Geometry check sheet. Reference: the model listing, model coordinates, mm. Face numbers are marked on the shaded views. A direction names the side the tool comes from. Coordinates: 2 decimals unless noted, no trailing zeros. Loops run counter-clockwise (first coordinate to the right, second up) from the corner with the lowest first, then second, coordinate; pieces in that order, holes last.
Solid Edge part; units mm, degrees
sketch "Sketch1" plane through (0, 0, 0) normal (0, -1, 0) x (1, 0, 0)
  line L0 (0, 25) -> (-95, 25)
  line L1 (-95, 25) -> (-95, 10)
  line L2 (-95, 10) -> (-45, 10)
  line L3 (-45, 10) -> (-45, -10)
  line L4 (-45, -10) -> (-95, -10)
  line L5 (-95, -10) -> (-95, -25)
  line L6 (-95, -25) -> (0, -25)
  arc A0 (0, 25) -> (0, -25) centre (0, 0) cw
  circle A1 centre (0, 0) radius 12.5
extrude "Protrusion1" add sketch "Sketch1" against normal blind 50
sketch "Sketch2" plane through (-47.5, 25, 25) normal (0, 0, 1) x (1, 0, 0)
  line L0 (-22.5, 25) -> (72.5, 25)
  line L1 (72.5, 25) -> (72.5, 10)
  line L2 (72.5, 10) -> (22.5, 10)
  line L3 (22.5, 10) -> (22.5, -10)
  line L4 (22.5, -10) -> (72.5, -10)
  line L5 (72.5, -10) -> (72.5, -25)
  line L6 (72.5, -25) -> (-22.5, -25)
  arc A0 (-22.5, -25) -> (-22.5, 25) centre (-22.5, 0) cw
  circle A1 centre (-22.5, 0) radius 12.5
extrude "ExtrudedProtrusion_2" add sketch "Sketch2" against normal blind 50
fillet "Round_2" radius 25 8 edges at (25, 42.5, 25) (25, 7.5, 25) (25, 42.5, -25) (25, 7.5, -25) (-95, 50, 17.5) (-95, 50, -17.5) (-95, 0, 17.5) (-95, 0, -17.5)
sketch "Sketch3" plane through (-22.5, 0, 0) normal (0, -1, 0) x (-1, 0, 0)
  circle A0 centre (-22.578, 0) radius 12.5
extrude "ExtrudedCutout_1" cut sketch "Sketch3" against normal blind 50
sketch "Sketch4" plane through (-47.5, 25, 25) normal (0, 0, 1) x (-1, 0, 0)
  circle A0 centre (22.5, 0) radius 12.5
extrude "ExtrudedCutout_2" cut sketch "Sketch4" against normal blind 50
sketch "Sketch5" plane through (-47.5, 25, 25) normal (0, 0, 1) x (-1, 0, 0)
  line L0 (-22.5, 10) -> (-72.5, 10)
  line L1 (-72.5, 10) -> (-72.5, -10)
  line L2 (-72.5, -10) -> (-22.5, -10)
  line L3 (-22.5, -10) -> (-22.5, 10)
extrude "ExtrudedCutout_3" cut sketch "Sketch5" against normal blind 50
sketch "Sketch6" plane through (-22.5, 0, 0) normal (0, -1, 0) x (0, 0, -1)
  line L0 (-10, -72.5) -> (10, -72.5)
  line L1 (10, -72.5) -> (10, -22.5)
  line L2 (10, -22.5) -> (-10, -22.5)
  line L3 (-10, -22.5) -> (-10, -72.5)
extrude "ExtrudedCutout_4" cut sketch "Sketch6" against normal blind 50
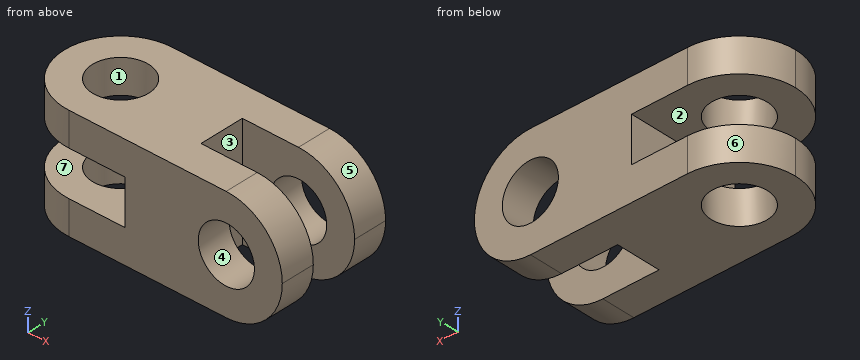
(1) Access from +Z, -Z, +X, -X, +Y, -Y to the whole of each face (thin tool, end or side, straight path). Record for the marked faces 1, 2 and 3.
Findings:
face 1: +Z, -Z
face 2: -X, +Y, -Y
face 3: +Z, -Z, +X
(2) Sectioned sample at D-D on x = -74. Record the cut outline in (y, z).
Findings:
outline: (0.32, -25) - (13.16, -25) - (13.16, -10) - (0.32, -10) - close; (0.32, 10) - (13.16, 10) - (13.16, 25) - (0.32, 25) - close; (36.84, -25) - (49.68, -25) - (49.68, -10) - (36.84, -10) - close; (36.84, 10) - (49.68, 10) - (49.68, 25) - (36.84, 25) - close
(3) Gauge pin test, flat ends, axial feed: pin 1 Ø6 at (y, z) = (11.5, -3.5) entering from +X; pin 2 Ø16 at (y, z) = (27.5, 1) entering from -X; pin 3 Ø12 at (y, z) = (14.5, -14.5) entering from -X. Record the tip position at first contact, or that the pin passes through.
Findings:
pin 1: stops at x = 25
pin 2: stops at x = -45
pin 3: stops at x = -94.59
(4) Sectioned sample at C-C on z = -5.5. Record the cut outline in (x, y), and give its area (3 significant figures).
Findings:
outline: (-45, 0) - (-11.15, 0) - (-11.15, 15) - (-25, 15) - (-25, 35) - (-11.15, 35) - (-11.15, 50) - (-45, 50) - close; (11.3, 0) - (24.39, 0) - (24.39, 15) - (11.3, 15) - close; (11.3, 35) - (24.39, 35) - (24.39, 50) - (11.3, 50) - close
area: 1,810 mm2
(5) Draft check along Z on the marked faces 4, 5, 6 and 7. Enter one of: +Z half, -Z half, draft (parallel to the pull), parting line (faces both ways), or undercut.
Findings:
face 4: undercut
face 5: +Z half
face 6: draft
face 7: undercut
(6) Scan lines: L1, parallel to Z at x = -74, y = 12.5; L2, parallel to Y at x = -14, z = 4; L3, parallel to X at y = 9.25, z = 0. Record each from-to range of solid material in increasing order.
Findings:
L1: z = -25 to -10, 10 to 25
L2: y = 0 to 15, 35 to 50
L3: x = -45 to -12.42, 12.58 to 25
(7) Sectioned sample at A-A on x = 7.5. Record the cut outline in (y, z), and give its area (3 significant figures).
Findings:
outline: (0, -23.85) - (15, -23.85) - (15, -10.06) - (0, -10.06) - close; (0, 10.06) - (15, 10.06) - (15, 23.85) - (0, 23.85) - close; (35, -23.85) - (50, -23.85) - (50, -10.06) - (35, -10.06) - close; (35, 10.06) - (50, 10.06) - (50, 23.85) - (35, 23.85) - close
area: 827 mm2
